```python
from build123d import *

# Parameters (mm, degrees)
SKETCH1_W           = 3.302
SKETCH1_H           = 38.1
BOSS_EXTRUDE1_DEPTH = 3.175
SKETCH2_R           = 0.627804746
CUT_EXTRUDE1_DEPTH  = 2.54


with BuildPart() as part:
    # Sketch1 → Boss-Extrude1 (new body)
    with BuildSketch(Plane(origin=(0, 0, 0), x_dir=(1, 0, 0), z_dir=(0, 1, 0))):
        with BuildLine():
            Line((-149.86, -55.88), (-149.86, 55.88))
            Line((-149.86, 55.88), (-111.76, 55.88))
            Line((-111.76, 55.88), (-111.76, 68.58))
            Line((-111.76, 68.58), (-86.36, 68.58))
            Line((-86.36, 68.58), (-86.36, 57.15))
            Line((-86.36, 57.15), (-83.058, 57.15))
            Line((-83.058, 57.15), (-83.058, 68.58))
            Line((-83.058, 68.58), (-1.651, 68.58))
            Line((-1.651, 68.58), (-1.651, 57.15))
            Line((-1.651, 57.15), (1.651, 57.15))
            Line((1.651, 57.15), (1.651, 68.58))
            Line((1.651, 68.58), (83.058, 68.58))
            Line((83.058, 68.58), (83.058, 57.15))
            Line((83.058, 57.15), (86.36, 57.15))
            Line((86.36, 57.15), (86.36, 68.58))
            Line((86.36, 68.58), (111.76, 68.58))
            Line((111.76, 68.58), (111.76, 55.88))
            Line((111.76, 55.88), (149.86, 55.88))
            ThreePointArc((149.86, 55.88), (205.74, 0), (149.86, -55.88))
            Line((149.86, -55.88), (111.76, -55.88))
            Line((111.76, -55.88), (111.76, -68.58))
            Line((111.76, -68.58), (86.36, -68.58))
            Line((86.36, -68.58), (86.36, -57.15))
            Line((86.36, -57.15), (83.058, -57.15))
            Line((83.058, -57.15), (83.058, -68.58))
            Line((83.058, -68.58), (1.651, -68.58))
            Line((1.651, -68.58), (1.651, -57.15))
            Line((1.651, -57.15), (-1.651, -57.15))
            Line((-1.651, -57.15), (-1.651, -68.58))
            Line((-1.651, -68.58), (-83.058, -68.58))
            Line((-83.058, -68.58), (-83.058, -57.15))
            Line((-83.058, -57.15), (-86.36, -57.15))
            Line((-86.36, -57.15), (-86.36, -68.58))
            Line((-86.36, -68.58), (-111.76, -68.58))
            Line((-111.76, -68.58), (-111.76, -55.88))
            Line((-111.76, -55.88), (-149.86, -55.88))
        make_face()
        Rectangle(SKETCH1_W, SKETCH1_H, mode=Mode.SUBTRACT)
        with Locations((-84.709, 0)):
            Rectangle(SKETCH1_W, SKETCH1_H, mode=Mode.SUBTRACT)
        with Locations((84.709, 0)):
            Rectangle(SKETCH1_W, SKETCH1_H, mode=Mode.SUBTRACT)
    extrude(amount=BOSS_EXTRUDE1_DEPTH)

    # Sketch2 → Cut-Extrude1 (cut)
    with BuildSketch(Plane.ZY.offset(149.86)):
        with Locations((0, 1.55575)):
            Circle(SKETCH2_R)
    extrude(amount=-CUT_EXTRUDE1_DEPTH, mode=Mode.SUBTRACT)


solid = part.part
```
CAD build for the part. Positions are in the model's coordinates, mm. Coordinates: 2 decimals unless noted, no trailing zeros. Order: outer loops, then holes, each group sorted by start corner. A loop starts at its lowest first (then second) coordinate and runs counter-clockwise, first axis right, second up.
(1) Drill centre lines: L1, parallel to X at y = 0.9, z = 2; L2, parallel to Y at x = -148.2, z = 0 (3 decimals); L3, parallel to X at y = 2.6, z = 7.5. Where is each one in solid material? Low to high.
Solution:
L1: x = -149.86 to -86.36, -83.06 to -1.65, 1.65 to 83.06, 86.36 to 205.7
L2: y = 0 to 0.928, 2.184 to 3.175
L3: x = -149.86 to -86.36, -83.06 to -1.65, 1.65 to 83.06, 86.36 to 205.23
(2) Saw through at A-A, the plane x = 127. Write the cut outline in (y, z) (3 decimals), and give its area (3 significant figures).
Solution:
outline: (0, -55.88) - (3.175, -55.88) - (3.175, 55.88) - (0, 55.88) - close
area: 355 mm2
(3) Pin check, flat tips, straight feed: pin 1 Ø1.6 at (x, y) = (136.5, 1.5) entering from -Z; pin 2 Ø6 at (x, z) = (149, 20.5) entering from -Y; pin 3 Ø1 at (x, y) = (-85.5, 1) entering from +Z; pin 4 Ø1 at (y, z) = (2, 62.5) entering from -X. Stop position of each tip, or through.
Solution:
pin 1: stops at z = -55.88
pin 2: stops at y = 0
pin 3: stops at z = 57.15
pin 4: stops at x = -111.76
